Build history of the part. All positions in model axes, mm. A direction names the side the tool comes from. Give positions to 0.01 mm unless a question says otherwise; leave off trailing zeros. Order: outer loops, then holes, each group sorted by start corner. A loop starts at its lowest first (then second) coordinate and runs counter-clockwise, first axis right, second up. Notation, with made-up numbers: M -5.75,-1.5 L -1.75,-1.5 A20 cw -1.75,28.5 Z; hole C 10.25,14.5 d11. An arc over 180 degrees is marked long. Use CSV: the item, a comma, the result in double quotes. Start each with the question number.
Item 1: Band-saw the part on B-B on y = -10.5. Write the cut outline in (x, z), plus the area to 3 significant figures.
Item 2: Wall check: line 1 along Y through (x, z) = (-3.5, -1); line 2 along Y through (x, z) = (-41, 28.5); line 3 along Z through (x, y) = (-2.5, 31.5). Give the ranges that are in metal, low to high.
Item 3: Which spindle directions (+Z, -Z, +X, -X, +Y, -Y) get a long thin tool onto all of the face, cutting with end or side? Do faces 5 (the cylindrical face through (3.2, 47.73, -2.03)), 6 (the cylindrical face through (-23.65, 31.3, 17.26)). Say none if no direction does.
Item 4: Pin check, flat tips, straight feed: P1, Ø1.5, axis at y = -7.5, z = 20, coming from the +X side; P2, Ø12, axis at x = -50, z = 7, coming from the +Y side; P3, Ø8, axis at x = -65.5, z = 28, coming from the +Y side; P4, Ø2.5, axis at x = -1.64, y = -27.7, coming from the +Z side. Stop position of each tip, or through.
Item 5: Band-saw the part on C-C on z = 2. Write the cut outline in (x, y).
Item 6: Two-plate mould, pull along X, no slides. Class faces 1 (the flat face through (-40, 6, 0)), 2 (the flat face through (-85.049, 5, -2)), 3 (the flat face through (-60, 36, 0)), 4 (the cylindrical face through (-3.71, 41.55, -1.97)): pulls with the +X half, pulls with the -X half, needs draft (parallel to the pull), parting line crosses it, or undercut.
Item 7: Band-saw the part on A-A on x = -11.5. Write the cut outline in (y, z).
from build123d import *

# Parameters (mm, degrees)
SKETCH1_W           = 170
SKETCH1_H           = 90
BOSS_EXTRUDE1_DEPTH = 5
SKETCH1_3_W         = 170
SKETCH1_3_H         = 90
SKETCH1_3_R         = 3
BOSS_EXTRUDE2_DEPTH = 10
SKETCH1_4_R         = 33.5
SKETCH1_4_R_2       = 30.5
BOSS_EXTRUDE3_DEPTH = 35
SKETCH1_7_R         = 33.5
BOSS_EXTRUDE4_DEPTH = 10
SKETCH3_W           = 78.746322612
SKETCH3_H           = 90
CUT_EXTRUDE3_DEPTH  = 10
SKETCH5_R           = 1.7
CUT_EXTRUDE4_DEPTH  = 10
SKETCH6_W           = 91.253677388
SKETCH6_H           = 90
CUT_EXTRUDE5_DEPTH  = 6
FILLET2_R           = 10


with BuildPart() as part:
    # Sketch1 → Boss-Extrude1 (new body)
    with BuildSketch(Plane.XY):
        with Locations((-0.049117786, 5.583941606)):
            Rectangle(SKETCH1_W, SKETCH1_H)
    extrude(amount=-BOSS_EXTRUDE1_DEPTH)

    # Sketch1<3> → Boss-Extrude2 (add)
    with BuildSketch(Plane.XY):
        with Locations((-0.049117786, 5.583941606)):
            Rectangle(SKETCH1_3_W, SKETCH1_3_H)
        with Locations((-77.306081152, -32.231283052)):
            Circle(SKETCH1_3_R, mode=Mode.SUBTRACT)
        with Locations((75.391495508, -30.531283052)):
            Circle(SKETCH1_3_R, mode=Mode.SUBTRACT)
        with Locations((75.391495508, 41.466476411)):
            Circle(SKETCH1_3_R, mode=Mode.SUBTRACT)
        with Locations((-77.306081152, 42.827274758)):
            Circle(SKETCH1_3_R, mode=Mode.SUBTRACT)
        with BuildLine():
            Line((-65.684201055, -34.416058394), (65.585965482, -34.416058394))
            ThreePointArc((65.585965482, -34.416058394), (70.80874659, -25.27392277), (79.950882214, -20.051141663))
            Line((79.950882214, -20.051141663), (79.950882214, 31.219024875))
            ThreePointArc((79.950882214, 31.219024875), (70.80874659, 36.441805982), (65.585965482, 45.583941606))
            Line((65.585965482, 45.583941606), (-65.684201055, 45.583941606))
            ThreePointArc((-65.684201055, 45.583941606), (-70.906982163, 36.441805982), (-80.049117786, 31.219024875))
            Line((-80.049117786, 31.219024875), (-80.049117786, -20.051141663))
            ThreePointArc((-80.049117786, -20.051141663), (-70.906982163, -25.27392277), (-65.684201055, -34.416058394))
        make_face(mode=Mode.SUBTRACT)
    extrude(amount=-BOSS_EXTRUDE2_DEPTH)

    # Sketch1<4> → Boss-Extrude3 (add)
    with BuildSketch(Plane.XY):
        with Locations((-40.049117786, 5.583941606)):
            Circle(SKETCH1_4_R)
        with Locations((-40.049117786, 5.583941606)):
            Circle(SKETCH1_4_R_2, mode=Mode.SUBTRACT)
    extrude(amount=BOSS_EXTRUDE3_DEPTH)

    # Sketch1<7> → Boss-Extrude4 (add)
    with BuildSketch(Plane.XY):
        with BuildLine():
            ThreePointArc((-65.684201055, -34.416058394), (-70.906982163, -25.27392277), (-80.049117786, -20.051141663))
            Line((-80.049117786, -20.051141663), (-80.049117786, 31.219024875))
            ThreePointArc((-80.049117786, 31.219024875), (-70.906982163, 36.441805982), (-65.684201055, 45.583941606))
            Line((-65.684201055, 45.583941606), (65.585965482, 45.583941606))
            ThreePointArc((65.585965482, 45.583941606), (70.80874659, 36.441805982), (79.950882214, 31.219024875))
            Line((79.950882214, 31.219024875), (79.950882214, -20.051141663))
            ThreePointArc((79.950882214, -20.051141663), (70.80874659, -25.27392277), (65.585965482, -34.416058394))
            Line((65.585965482, -34.416058394), (-65.684201055, -34.416058394))
        make_face()
        with Locations((-40.049117786, 5.583941606)):
            Circle(SKETCH1_7_R, mode=Mode.SUBTRACT)
    extrude(amount=-BOSS_EXTRUDE4_DEPTH)

    # Sketch3 → Cut-Extrude3 (cut)
    with BuildSketch(Plane.XY):
        with Locations((45.577720908, 5.583941606)):
            Rectangle(SKETCH3_W, SKETCH3_H)
    extrude(amount=-CUT_EXTRUDE3_DEPTH, mode=Mode.SUBTRACT)

    # Sketch5 → Cut-Extrude4 (cut)
    with BuildSketch(Plane.XY):
        with Locations((-76.777993439, 43.20743885)):
            Circle(SKETCH5_R)
        with Locations((-3.340612715, 43.20743885)):
            Circle(SKETCH5_R)
        with Locations((-76.777993439, -29.399888528)):
            Circle(SKETCH5_R)
        with Locations((-1.640612715, -27.699888528)):
            Circle(SKETCH5_R)
    extrude(amount=-CUT_EXTRUDE4_DEPTH, mode=Mode.SUBTRACT)

    # Sketch6 → Cut-Extrude5 (cut)
    with BuildSketch(Plane(origin=(0, 0, -10), x_dir=(-1, 0, 0), z_dir=(0, 0, -1))):
        with Locations((39.422279092, 5.583941606)):
            Rectangle(SKETCH6_W, SKETCH6_H)
    extrude(amount=-CUT_EXTRUDE5_DEPTH, mode=Mode.SUBTRACT)

    # Fillet2
    fillet2_edges = [part.edges().sort_by_distance(p)[0] for p in [
        (6.204559602, -39.416058394, -2),
        (6.204559602, 50.583941606, -2),
        (-85.049117786, -39.416058394, -2),
        (-85.049117786, 50.583941606, -2),
    ]]
    fillet(fillet2_edges, radius=FILLET2_R)


solid = part.part
Model answer:
1,outline,"M -85.05,-4 L 6.2,-4 L 6.2,0 L -10.66,0 L -10.66,35 L -14.13,35 L -14.13,0 L -65.96,0 L -65.96,35 L -69.44,35 L -69.44,0 L -85.05,0 Z"
1,area,"608 mm^2"
2,line 1,"y = -39.41 to 41.51, 44.9 to 50.58"
2,line 2,"y = -27.9 to -24.9, 36.07 to 39.07"
2,line 3,"z = -4 to 0"
3,face 5,"+Z, -Z, +X, +Y"
3,face 6,"+Z"
4,P1,"stops at x = -8.9"
4,P2,"stops at y = 38.85"
4,P3,"stops at y = 31.32"
4,P4,"passes through"
5,outline,"C -40.05,5.58 d67; hole C -40.05,5.58 d61"
6,face 1,"undercut"
6,face 2,"pulls with the -X half"
6,face 3,"needs draft"
6,face 4,"undercut"
7,outline,"M -39.42,-4 L 50.58,-4 L 50.58,0 L 23.11,0 L 23.11,35 L 16.32,35 L 16.32,0 L -5.15,0 L -5.15,35 L -11.94,35 L -11.94,0 L -39.42,0 Z"
